from build123d import *

# Parameters (mm, degrees)
F0_R     = 1.25
F0_R_2   = 3
F0_R_3   = 3.25
F1_DEPTH = 2.4
F2_DEPTH = 1.4
F3_SIZE  = 0.2
F4_SIZE  = 0.2


with BuildPart() as f1:
    # F0 (on Top) → F1 (new body)
    with BuildSketch(Plane.XY):
        with BuildLine():
            ThreePointArc((8.61, 0.26), (7.4384271247, 3.0884271247), (4.61, 4.26))
            Line((4.61, 4.26), (-4.61, 4.26))
            ThreePointArc((-4.61, 4.26), (-7.4384271247, 3.0884271247), (-8.61, 0.26))
            Line((-8.61, 0.26), (-8.61, -4.26))
            Line((-8.61, -4.26), (8.61, -4.26))
            Line((8.61, -4.26), (8.61, 0.26))
        make_face()
        with Locations((-6.1, 0)):
            Circle(F0_R, mode=Mode.SUBTRACT)
        Circle(F0_R_2, mode=Mode.SUBTRACT)
        with Locations((6.1, 0)):
            Circle(F0_R, mode=Mode.SUBTRACT)
        with BuildLine():
            Line((8.61, -11.06), (8.61, -4.26))
            Line((8.61, -4.26), (-8.61, -4.26))
            Line((-8.61, -4.26), (-8.61, -11.06))
            ThreePointArc((-8.61, -11.06), (-7.4384271247, -13.8884271247), (-4.61, -15.06))
            Line((-4.61, -15.06), (4.61, -15.06))
            ThreePointArc((4.61, -15.06), (7.4384271247, -13.8884271247), (8.61, -11.06))
        make_face()
        with Locations((-6.1, -10.55)):
            Circle(F0_R, mode=Mode.SUBTRACT)
        with Locations((0, -10.55)):
            Circle(F0_R_3, mode=Mode.SUBTRACT)
        with Locations((6.1, -10.55)):
            Circle(F0_R, mode=Mode.SUBTRACT)
        Circle(F0_R_2)
    extrude(amount=-F1_DEPTH)

    # F0 (on Top) → F2 (join)
    with BuildSketch(Plane.XY):
        Circle(F0_R_2)
    extrude(amount=F2_DEPTH)

    # F3
    f3_edges = [f1.edges().sort_by_distance(p)[0] for p in [
        (7.438427, 3.088427, -2.4),
        (0, 4.26, -2.4),
        (-7.438427, 3.088427, -2.4),
        (-8.61, -5.4, -2.4),
        (-7.438427, -13.888427, -2.4),
        (0, -15.06, -2.4),
        (7.438427, -13.888427, -2.4),
        (8.61, -5.4, -2.4),
        (-7.35, 0, -2.4),
        (4.85, 0, -2.4),
        (4.85, -10.55, -2.4),
        (-7.35, -10.55, -2.4),
        (-3.25, -10.55, -2.4),
    ]]
    chamfer(f3_edges, length=F3_SIZE)

    # F4
    f4_edges = [f1.edges().sort_by_distance(p)[0] for p in [
        (-3, 0, 1.4),
    ]]
    chamfer(f4_edges, length=F4_SIZE)


solid = f1.part
The model under review builds one solid part; all positions refer to its coordinate system, in mm. Round coordinates to 2 decimals unless told otherwise and drop trailing zeros. Order: outer loops, then holes, each group sorted by start corner. A loop starts at its lowest first (then second) coordinate and runs counter-clockwise, first axis right, second up. Notation, with made-up numbers: (-28, 32) -> (19, 32) arc R25 ccw to (19, 62) -> close; hole circle Ø1 at (48.25, -36). An arc over 180 degrees is marked (long way). Use CSV: the item, a comma, the result in double quotes. Start each with the question number.
(1) Consider section A-A on y = -10.55. Write out the cut boundary in (x, z), and give its area (3 significant figures).
(2) Mouldability with a two-part tool opening along Y and no side actions: class faces 1 (the face through (-7.469, -13.857, -1.085)), 2 (the face through (-3, 0, 1)), 3 (the face through (7.29, 0.38, -1.08)), 4 (the face through (-7.35, 0.05, -1.08)) as pulls with the +Y half, pulls with the -Y half, needs draft (parallel to the pull), parting line crosses it, or undercut.
(3) Insertion check: pin 1 (3 mm diameter, centred on x = 6.1, y = -10.55, fed in from +Z); pin 2 (2 mm diameter, centred on x = -6.1, y = 0, fed in from +Z); pin 3 (1.5 mm diameter, centred on x = -6.5, z = 0, fed in from -Y). Each pin has a flat end and moves straight along its axis. Give the tip position at first contact, or say it passes through.
(4) Consider section D-D on x = -5.75. State how many separate pieces and enclosed holes the cut face has, and give its area (3 significant figures).
(5) Consider section B-B on y = 0. Write out the cut boundary in (x, z), and give its area (3 significant figures).
(6) Consider section C-C on z = -0.6. Write out the cut boundary in (x, y), and give its area (3 significant figures).
(7) Wall thickness on probe 1 along Y at (x, z) = (0, -0.6); probe 2 along Y at (x, z) = (6.1, -0.6); probe 3 along X at (y, z) = (1.5, -1.3): over which ranges is each line inside the solid? List them lowest first. Write a range as from..to.
Responses:
1,outline,"(-8.61, -2.2) -> (-8.41, -2.4) -> (-7.55, -2.4) -> (-7.35, -2.2) -> (-7.35, 0) -> (-8.61, 0) -> close; (-4.85, -2.2) -> (-4.65, -2.4) -> (-3.45, -2.4) -> (-3.25, -2.2) -> (-3.25, 0) -> (-4.85, 0) -> close; (3.25, -2.2) -> (3.45, -2.4) -> (4.65, -2.4) -> (4.85, -2.2) -> (4.85, 0) -> (3.25, 0) -> close; (7.35, -2.2) -> (7.55, -2.4) -> (8.41, -2.4) -> (8.61, -2.2) -> (8.61, 0) -> (7.35, 0) -> close"
1,area,"13.6 mm²"
2,face 1,"pulls with the -Y half"
2,face 2,"parting line crosses it"
2,face 3,"undercut"
2,face 4,"undercut"
3,pin 1,"z = 0"
3,pin 2,"through"
3,pin 3,"y = -14.89"
4,separate pieces,"3"
4,enclosed holes,"0"
4,area,"33.9 mm²"
5,outline,"(-8.61, -2.2) -> (-8.41, -2.4) -> (-7.55, -2.4) -> (-7.35, -2.2) -> (-7.35, 0) -> (-8.61, 0) -> close; (-4.85, -2.2) -> (-4.65, -2.4) -> (4.65, -2.4) -> (4.85, -2.2) -> (4.85, 0) -> (3, 0) -> (3, 1.2) -> (2.8, 1.4) -> (-2.8, 1.4) -> (-3, 1.2) -> (-3, 0) -> (-4.85, 0) -> close; (7.35, -2.2) -> (7.55, -2.4) -> (8.41, -2.4) -> (8.61, -2.2) -> (8.61, 0) -> (7.35, 0) -> close"
5,area,"37.6 mm²"
6,outline,"(-8.61, -11.06) arc R4 ccw to (-4.61, -15.06) -> (4.61, -15.06) arc R4 ccw to (8.61, -11.06) -> (8.61, 0.26) arc R4 ccw to (4.61, 4.26) -> (-4.61, 4.26) arc R4 ccw to (-8.61, 0.26) -> close; hole circle Ø2.5 at (-6.1, -10.55); hole circle Ø2.5 at (-6.1, 0); hole circle Ø6.5 at (0, -10.55); hole circle Ø2.5 at (6.1, -10.55); hole circle Ø2.5 at (6.1, 0)"
6,area,"266 mm²"
7,probe 1,"-15.06..-13.8, -7.3..4.26"
7,probe 2,"-14.77..-11.8, -9.3..-1.25, 1.25..3.97"
7,probe 3,"-8.41..8.41"
